from build123d import *

# Parameters (mm, degrees)
F1_DEPTH = 12.7
F3_DEPTH = 1.27
F5_DEPTH = 2.54


with BuildPart() as f1:
    # F0 (on Top) → F1 (new body)
    with BuildSketch(Plane.XY):
        Polygon((14.664697, 0), (7.332348, 12.7), (-7.332348, 12.7), (-14.664697, 0), (-7.332348, -12.7), (7.332348, -12.7), align=None)
    extrude(amount=F1_DEPTH)

    # F2 (on face) → F3 (cut)
    with BuildSketch(Plane.XY.offset(12.7)):
        Polygon((3.175, 10.16), (-3.175, 10.16), (-3.175, 3.175), (-10.16, 3.175), (-10.16, -3.175), (-3.175, -3.175), (-3.175, -10.16), (3.175, -10.16), (3.175, -3.175), (10.16, -3.175), (10.16, 3.175), (3.175, 3.175), align=None)
    extrude(amount=-F3_DEPTH, mode=Mode.SUBTRACT)

    # F4 (on face) → F5 (cut)
    with BuildSketch(Plane.XY.offset(11.43)):
        with BuildLine():
            Line((2.54, 0.440925), (2.54, 1.016))
            ThreePointArc((2.54, 1.016), (0, 3.556), (-2.54, 1.016))
            Line((-2.54, 1.016), (-2.54, 0.440925))
            ThreePointArc((-2.54, 0.440925), (-2.343144, -0.959542), (-1.767831, -2.25147))
            Line((-1.767831, -2.25147), (0, -5.08))
            Line((0, -5.08), (1.767831, -2.25147))
            ThreePointArc((1.767831, -2.25147), (2.343144, -0.959542), (2.54, 0.440925))
        make_face()
    extrude(amount=-F5_DEPTH, mode=Mode.SUBTRACT)


solid = f1.part
The model under review builds one solid part; all positions refer to its coordinate system, in mm. A direction names the side the tool comes from. Round coordinates to 2 decimals unless told otherwise and drop trailing zeros. Order: outer loops, then holes, each group sorted by start corner. A loop starts at its lowest first (then second) coordinate and runs counter-clockwise, first axis right, second up. Notation, with made-up numbers: (3.25, 6) - (12.25, 6) arc R19 ccw to (12.25, 16) - close; hole circle Ø3 at (15, 41). An arc over 180 degrees is marked (long way). Use one line per item in the form item = value.
Q1. Mouldability with a two-part tool opening along Y and no side actions: class faces 3 (the flat face through (-7, -3.175, 12)), 4 (the flat face through (-10.947, 6.439, 6.261)), 5 (the flat face through (-3.175, 7, 12)), 6 (the flat face through (10.947, -6.439, 6.261)) as pulls with the +Y half, pulls with the -Y half, needs draft (parallel to the pull), parting line crosses it, or undercut.
Response values:
face_3 = undercut
face_4 = pulls with the +Y half
face_5 = undercut
face_6 = pulls with the -Y half
Q2. Clearance check with flat-ended pins moving along their axes: P1, Ø0.6, axis at y = -5, z = 12, coming from the +X side; P2, Ø0.6, axis at y = 1, z = 9.5, coming from the -X side; P3, Ø3, axis at y = 0, z = 8, coming from the +X side. State where each tip first meets the part, or that it passes through.
Response values:
P1 = 11.95
P2 = -14.26
P3 = 14.66
Q3. Add section B-B on x = -0.5. Give the boundary of the cut face in (y, z).
Response values:
outline = (-12.7, 0) - (12.7, 0) - (12.7, 12.7) - (10.16, 12.7) - (10.16, 11.43) - (3.51, 11.43) - (3.51, 8.89) - (-4.28, 8.89) - (-4.28, 11.43) - (-10.16, 11.43) - (-10.16, 12.7) - (-12.7, 12.7) - close
Q4. To check wall thickness, follow line 1 (Z direction, x = 3, y = 8.5); line 2 (Y direction, x = 2.25, z = 11.5); line 3 (X direction, y = -6, z = 11.5) (3 decimals). State the ranges of each line that lie inside material, in increasing order.
Response values:
line_1 = 0 to 11.43
line_2 = -12.7 to -10.16, 10.16 to 12.7
line_3 = -11.201 to -3.175, 3.175 to 11.201
Q5. Add section D-D on x = 9.5. Give the boundary of the cut face in (y, z) (3 decimals), then the cut area to 3 significant figures.
Response values:
outline = (-8.946, 0) - (8.946, 0) - (8.946, 12.7) - (3.175, 12.7) - (3.175, 11.43) - (-3.175, 11.43) - (-3.175, 12.7) - (-8.946, 12.7) - close
area = 219 mm^2
Q6. Add section A-A on z = 9.5. Give the boundary of the cut face in (x, y).
Response values:
outline = (-14.66, 0) - (-7.33, -12.7) - (7.33, -12.7) - (14.66, 0) - (7.33, 12.7) - (-7.33, 12.7) - close; hole (-2.54, 0.44) arc R5.08 ccw to (-1.77, -2.25) - (0, -5.08) - (1.77, -2.25) arc R5.08 ccw to (2.54, 0.44) - (2.54, 1.02) arc R2.54 ccw to (-2.54, 1.02) - close
Q7. Tool access review of faces 1 (the flat face through (-10.16, 0, 12)), 2 (the flat face through (0, -12.7, 6)): name each direction out of +Z, -Z, +X, -X, +Y, -Y from which nothing blocks a thin tool from reaching the whole face with its end or side.
Response values:
face_1 = +Z
face_2 = +Z, -Z, +X, -X, -Y
Q8. Add section C-C on y = -7.25. Give the boundary of the cut face in (x, z) (3 decimals).
Response values:
outline = (-10.479, 0) - (10.479, 0) - (10.479, 12.7) - (3.175, 12.7) - (3.175, 11.43) - (-3.175, 11.43) - (-3.175, 12.7) - (-10.479, 12.7) - close
